Geometry: see drawing. Coordinates: mm, zero at the bounding-box minimum. A direction names the side the tool comes from. Give positions to 0.01 mm unless a question says otherwise; leave off trailing zeros. Order: outer loops, then holes, each group sorted by start corner. A loop starts at its lowest first (then second) coordinate and runs counter-clockwise, first axis right, second up. Notation, with made-up numbers: (35, 38) - (39, 38) arc R26 ccw to (39, 53) - close; hole circle Ø11 at (0.5, 26). An arc over 180 degrees is marked (long way). Write each question's results on one line, items separated by ' | '. Start each with the question number.
Item 1: Contact query for flat-ended pins moving along their axis: pin 1 Ø1.5 at (x, y) = (12, 10.5) entering from -Z; pin 2 Ø6 at (x, y) = (4, 13) entering from -Z; pin 3 Ø1 at (y, z) = (13.5, 3) entering from +X. Output: stop coordinate, or through.
Item 2: Line query: line 1 along X through (y, z) = (8.25, 8); line 2 along Y through (x, z) = (10, 1.25); line 3 along Z through (x, y) = (8, 5). Output: solid intervals per line, ascending.
Item 3: Section D-D on y = 8.5. Output: boundary loops of the cut face in (x, z).
Item 4: Set-up query: the marked faces 1 and 2. Return all of +Z, -Z, +X, -X, +Y, -Y with unobstructed straight access to the full face (end or side cutting, diameter ignored); none if empty.
Item 5: Section C-C on y = 14.75. Output: boundary loops of the cut face in (x, z), and give its area (3 significant figures).
Item 6: Section B-B on x = 8. Output: boundary loops of the cut face in (y, z), and give its area (3 significant figures).
Item 7: Section A-A on z = 8. Output: boundary loops of the cut face in (x, y).
Item 8: Mould query, pull axis X, two halves, no side actions, for the marked faces 3, 4 and 5. Classes: released by +X, released by -X, zero draft, split by the parting line, or undercut.
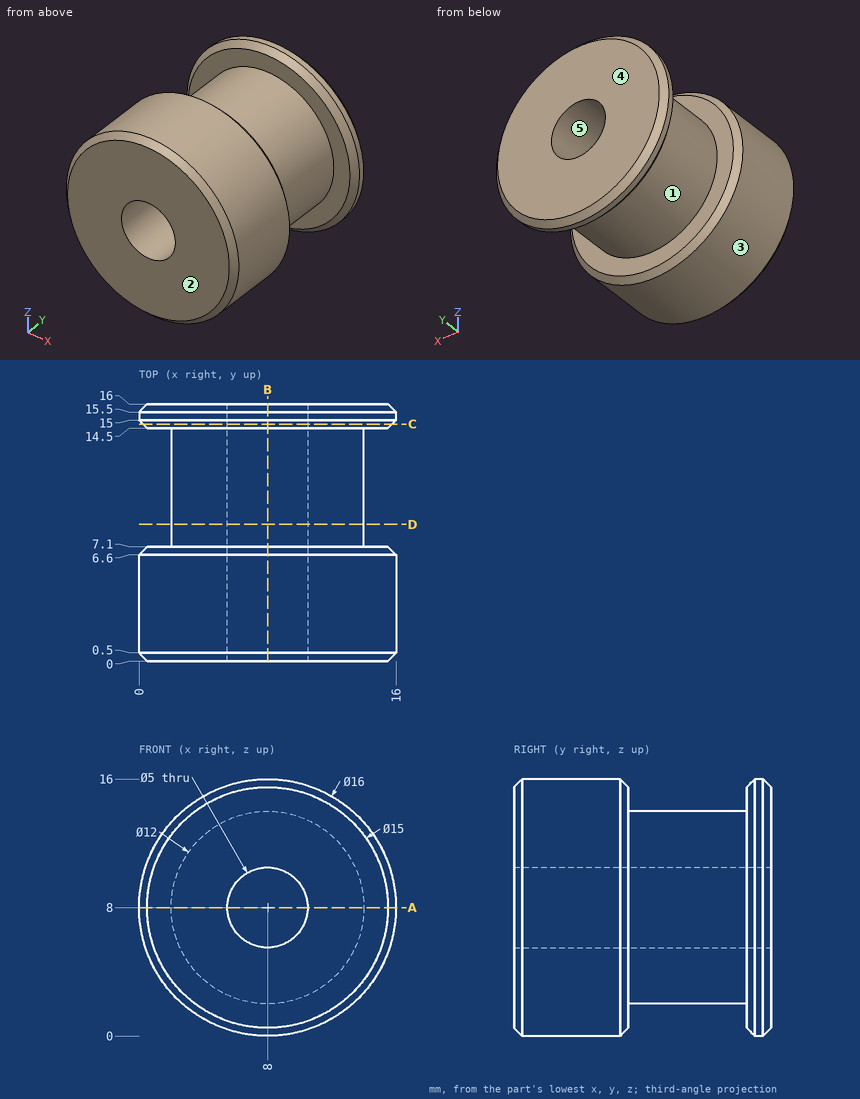
Evaluation:
1) pin 1: stops at z = 2.96 | pin 2: stops at z = 0.2 | pin 3: stops at x = 11.97
2) line 1: x = 2 to 5.5, 10.5 to 14 | line 2: y = 0 to 7.1, 14.5 to 16 | line 3: z = 0 to 5.5, 10.5 to 16
3) outline: circle Ø12 at (8, 8); hole circle Ø5 at (8, 8)
4) face 1: none | face 2: +Z, -Z, +X, -X, -Y
5) outline: circle Ø15.5 at (8, 8); hole circle Ø5 at (8, 8) | area: 169 mm^2
6) outline: (0, 0.5) - (0.5, 0) - (6.6, 0) - (7.1, 0.5) - (7.1, 2) - (14.5, 2) - (14.5, 0.5) - (15, 0) - (15.5, 0) - (16, 0.5) - (16, 5.5) - (0, 5.5) - close; (0, 10.5) - (16, 10.5) - (16, 15.5) - (15.5, 16) - (15, 16) - (14.5, 15.5) - (14.5, 14) - (7.1, 14) - (7.1, 15.5) - (6.6, 16) - (0.5, 16) - (0, 15.5) - close | area: 145 mm^2
7) outline: (0, 0.5) - (0.5, 0) - (5.5, 0) - (5.5, 16) - (0.5, 16) - (0, 15.5) - (0, 15) - (0.5, 14.5) - (2, 14.5) - (2, 7.1) - (0.5, 7.1) - (0, 6.6) - close; (10.5, 0) - (15.5, 0) - (16, 0.5) - (16, 6.6) - (15.5, 7.1) - (14, 7.1) - (14, 14.5) - (15.5, 14.5) - (16, 15) - (16, 15.5) - (15.5, 16) - (10.5, 16) - close
8) face 3: split by the parting line | face 4: zero draft | face 5: undercut
